from build123d import *

# Parameters (mm, degrees)
SKETCH1_W           = 77
SKETCH1_H           = 12
BOSS_EXTRUDE1_DEPTH = 10
SKETCH2_R           = 1.25
CUT_EXTRUDE1_DEPTH  = 12
SKETCH3_W           = 77
SKETCH3_H           = 20
BOSS_EXTRUDE2_DEPTH = 5
SKETCH4_W           = 30
SKETCH4_H           = 6
CUT_EXTRUDE2_DEPTH  = 10
SKETCH5_W           = 78
SKETCH5_H           = 5
CUT_EXTRUDE3_DEPTH  = 5
CUT_EXTRUDE4_DEPTH  = 12
SKETCH8_W           = 77
SKETCH8_H           = 5
BOSS_EXTRUDE3_DEPTH = 10


with BuildPart() as part:
    # Sketch1 → Boss-Extrude1 (new body)
    with BuildSketch(Plane.XY):
        with Locations((38.5, 6)):
            Rectangle(SKETCH1_W, SKETCH1_H)
    extrude(amount=BOSS_EXTRUDE1_DEPTH)

    # Sketch2 → Cut-Extrude1 (cut)
    with BuildSketch(Plane(origin=(77, 0, 0), x_dir=(0, 0, -1), z_dir=(1, 0, 0))):
        with Locations((-5, 3)):
            Circle(SKETCH2_R)
        with Locations((-5, 9)):
            Circle(SKETCH2_R)
    extrude(amount=-CUT_EXTRUDE1_DEPTH, mode=Mode.SUBTRACT)

    # Sketch3 → Boss-Extrude2 (add)
    with BuildSketch(Plane(origin=(0, 12, 0), x_dir=(1, 0, 0), z_dir=(0, 1, 0))):
        with Locations((38.5, -10)):
            Rectangle(SKETCH3_W, SKETCH3_H)
    boss_extrude2 = extrude(amount=BOSS_EXTRUDE2_DEPTH)

    # Mirror2: Boss-Extrude2 across plane
    add(boss_extrude2.mirror(Plane(origin=(0, 6, 0), x_dir=(0, 0, 1), z_dir=(0, -1, 0))))

    # Sketch4 → Cut-Extrude2 (cut)
    with BuildSketch(Plane(origin=(0, 0, 0), x_dir=(-1, 0, 0), z_dir=(0, 0, -1))):
        with Locations((-38.5, 9)):
            Rectangle(SKETCH4_W, SKETCH4_H)
        with Locations((-38.5, 3)):
            Rectangle(SKETCH4_W, SKETCH4_H)
    extrude(amount=-CUT_EXTRUDE2_DEPTH, mode=Mode.SUBTRACT)

    # Sketch5 → Cut-Extrude3 (cut)
    with BuildSketch(Plane.XY.offset(20)):
        with Locations((38.5, -2.5)):
            Rectangle(SKETCH5_W, SKETCH5_H)
    extrude(amount=-CUT_EXTRUDE3_DEPTH, mode=Mode.SUBTRACT)

    # Sketch6 → Cut-Extrude4 (cut)
    with BuildSketch(Plane.ZY):
        with BuildLine():
            ThreePointArc((3.75, 6), (5, 4.75), (6.25, 6))
            Line((6.25, 6), (3.75, 6))
        make_face()
        with BuildLine():
            Line((3.75, 6), (6.25, 6))
            ThreePointArc((6.25, 6), (5, 7.25), (3.75, 6))
        make_face()
    extrude(amount=-CUT_EXTRUDE4_DEPTH, mode=Mode.SUBTRACT)

    # Sketch8 → Boss-Extrude3 (add)
    with BuildSketch(Plane.XY.offset(20)):
        with Locations((38.5, 14.5)):
            Rectangle(SKETCH8_W, SKETCH8_H)
    extrude(amount=BOSS_EXTRUDE3_DEPTH)


solid = part.part
The listing builds one solid part. Answer for the finished solid, in the listing's coordinates (mm). A direction names the side the tool comes from. Round coordinates to 2 decimals unless told otherwise and drop trailing zeros. Write each loop counter-clockwise with the first axis right and the second up, starting at its lowest first coordinate (ties: lowest second). Pieces come first, ordered by that corner, then holes. Notation, with made-up numbers: (-21.5, 58.5) - (1.5, 58.5) arc R31 cw to (1.5, 94.5) - close; hole circle Ø2 at (-18, -16). An arc over 180 degrees is marked (long way). Use a Markdown table: item, result. Add a question column.
1. The part is cut by section B-B (x = 26.5). Write down the section's boundary in (y, z).
2. The part is cut by section D-D (x = 71). Write down the section's boundary in (y, z).
3. A tool of negligible diameter and unlimited length cuts with its end or side. For faces 5 (the face through (5.92, 4.78, 4.73)), 6 (the face through (38, 0, 9)), 7 (the face through (71.08, 10.24, 5.16)), from which of +Z, -Z, +X, -X, +Y, -Y can it reach the whole face along a straight path? Write none if from no direction.
4. Flat-ended cylindrical pins translate along their axes: P1, Ø13, axis at x = 12, y = 3, coming from the +Z side; P2, Ø1.2, axis at y = 3, z = 5.5, coming from the +X side; P3, Ø1.5, axis at x = 20.5, z = 27, coming from the -Y side. Find the tip coordinate at first contact, or state that the pin passes through.
5. The part is cut by section A-A (y = 11.25). Write down the section's boundary in (x, z), and give its area (3 significant figures).
6. Consider line 1 (Y direction, x = 73, z = 5); line 2 (Y direction, x = 41, z = 1.5); line 3 (Y direction, x = 9, z = 5). Determine where each line is inside the solid, lowest interval first.
7. For a pull along Z with two mould halves and no side action, classify faces 1 (the face through (65, 6, 10)), 2 (the face through (0, 8, 8)), 3 (the face through (12, 6, 5)), 4 (the face through (65, 3, 5)) as +Z half, -Z half, draft (parallel to the pull), parting line (faces both ways), or undercut.
8. The part is cut by section C-C (z = 5). Write down the section's boundary in (x, y).
Reported:
| question | item | result |
|---|---|---|
| 1 | outline | (-5, 0) - (0, 0) - (0, 15) - (-5, 15) - close; (12, 0) - (17, 0) - (17, 30) - (12, 30) - close |
| 2 | outline | (-5, 0) - (17, 0) - (17, 30) - (12, 30) - (12, 10) - (0, 10) - (0, 15) - (-5, 15) - close; hole circle Ø2.5 at (3, 5); hole circle Ø2.5 at (9, 5) |
| 3 | face 5 | -X |
| 3 | face 6 | +Z |
| 3 | face 7 | +X |
| 4 | P1 | z = 15 |
| 4 | P2 | x = 65 |
| 4 | P3 | y = 12 |
| 5 | outline | (0, 0) - (23.5, 0) - (23.5, 10) - (0, 10) - close; (53.5, 0) - (77, 0) - (77, 10) - (53.5, 10) - close |
| 5 | area | 470 mm^2 |
| 6 | line 1 | -5 to 1.75, 4.25 to 7.75, 10.25 to 17 |
| 6 | line 2 | -5 to 0, 12 to 17 |
| 6 | line 3 | -5 to 4.75, 7.25 to 17 |
| 7 | face 1 | +Z half |
| 7 | face 2 | draft |
| 7 | face 3 | undercut |
| 7 | face 4 | undercut |
| 8 | outline | (0, -5) - (77, -5) - (77, 1.75) - (65, 1.75) - (65, 4.25) - (77, 4.25) - (77, 7.75) - (65, 7.75) - (65, 10.25) - (77, 10.25) - (77, 17) - (0, 17) - (0, 7.25) - (12, 7.25) - (12, 4.75) - (0, 4.75) - close; hole (23.5, 0) - (53.5, 0) - (53.5, 12) - (23.5, 12) - close |
